The model under review builds one solid part; all positions refer to its coordinate system, in mm. Round coordinates to 2 decimals unless told otherwise and drop trailing zeros. Answer as a JSON object with one key per item and string values. Group by question number.
1) Insertion check: pin 1 Ø8 at (y, z) = (4, 57) entering from -X; pin 2 Ø3 at (y, z) = (4, 68) entering from +X; pin 3 Ø4 at (y, z) = (3, 47.5) entering from -X. Each pin has a flat end and moves straight along its axis. Give the tip position at first contact, or say it passes through.
2) To check wall thickness, follow probe 1 along Z at (x, y) = (0.5, -13); probe 2 along Z at (x, y) = (-1.5, 2); probe 3 along Z at (x, y) = (0, -3.5). State the ranges of each line that lie inside material, in increasing order. Write a range as [from, to].
3) We need section A-A, the plane x = 19. Count the separate pieces of the cut face and the enclosed holes in it, then the cut area to 3 significant figures.
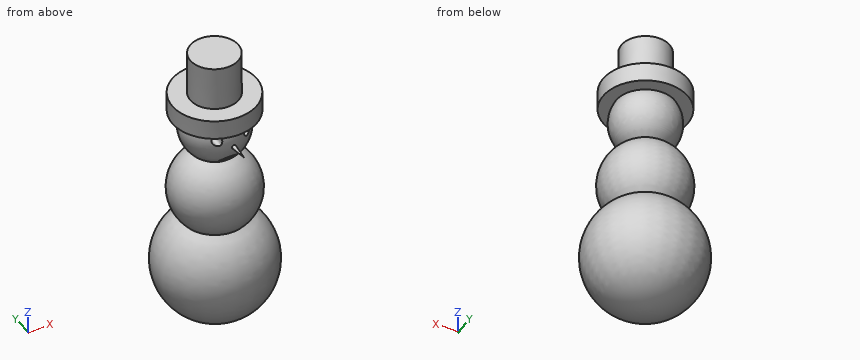
from build123d import *

# Parameters (mm, degrees)
F4_R     = 2.9313934917
F6_DEPTH = 25.4


with BuildPart() as f1:
    # F0 (on Front) → F1 (revolve)
    with BuildSketch(Plane.XZ):
        with BuildLine():
            ThreePointArc((-8.6470126601, 59.8095870837), (-21.4016690603, 44.0535851857), (-15.695191047, 24.6018766648))
            ThreePointArc((-15.695191047, 24.6018766648), (-28.0136061915, -8.1749144079), (0, -29.1820382673))
            Line((0, -29.1820382673), (-0.3967727534, 114.0140891075))
            Line((-0.3967727534, 114.0140891075), (-12.4211851507, 114.0140891075))
            Line((-12.4211851507, 114.0140891075), (-12.4211851507, 92.0014604926))
            Line((-12.4211851507, 92.0014604926), (-21.4189756662, 92.0014604926))
            Line((-21.4189756662, 92.0014604926), (-21.4189756662, 82.3283791542))
            Line((-21.4189756662, 82.3283791542), (-14.9194911479, 82.3283791542))
            ThreePointArc((-14.9194911479, 82.3283791542), (-16.2978226924, 69.8114756975), (-8.6470126601, 59.8095870837))
        make_face()
    revolve(axis=Axis((-0.1983863767, 0, 42.4160254201), (0.0027708237, 0, -0.9999961613)))

    # F4 (on Front) → F5 section 0
    with BuildSketch(Plane.XZ, mode=Mode.PRIVATE) as f5_s0:
        with Locations((0, 72.6552978158)):
            Circle(F4_R)
    loft([Vertex(0, -25.4, 72.6552978158), f5_s0.sketch])

    # F3 (on offset) → F6 (cut)
    with BuildSketch(Plane.XZ.offset(25.4)):
        with BuildLine():
            add(Edge.make_bspline(
                [(-8.0269714817, 79.5348510146), (-8.6846337437, 79.4264052352), (-9.8414942897, 78.1450545351), (-9.497142748, 75.3585343357), (-5.8915269462, 74.1267113958), (-5.1057227017, 77.4839777864), (-5.9214182567, 78.8940297376), (-7.3670372691, 79.6436714293), (-8.0269714817, 79.5348510146)],
                knots=[0, 0, 0, 0, 0.1593701812, 0.3340862186, 0.5188256822, 0.6983768822, 0.8400792609, 1, 1, 1, 1], degree=3))
        make_face()
        with BuildLine():
            add(Edge.make_bspline(
                [(8.3799511194, 78.3284604549), (7.624080444, 78.6857899226), (5.8447857804, 78.4029369239), (5.6907424207, 76.3172160457), (7.506583602, 73.9429964977), (10.3601830594, 76.0452757725), (9.1859243667, 77.9474455529), (8.3799511194, 78.3284604549)],
                knots=[0, 0, 0, 0, 0.1981616253, 0.3732706853, 0.5804624626, 0.7887033142, 1, 1, 1, 1], degree=3))
        make_face()
        with BuildLine():
            Line((3.1171578952, 62.8545942359), (4.2782197706, 63.3692070842))
            ThreePointArc((4.2782197706, 63.3692070842), (-0.4267061595, 66.4302188327), (-5.1316320896, 63.3692070842))
            Line((-5.1316320896, 63.3692070842), (-3.9705702142, 62.8545942359))
            ThreePointArc((-3.9705702142, 62.8545942359), (-0.4267061595, 65.1602223516), (3.1171578952, 62.8545942359))
        make_face()
    extrude(amount=-F6_DEPTH, mode=Mode.SUBTRACT)


solid = f1.part
Here are the results:
{
 "1": {"pin 1": "stops at x = -17", "pin 2": "stops at x = 15.24", "pin 3": "stops at x = -20.9"},
 "2": {"probe 1": "z = [-26.08, 57.14], [63.91, 65.05], [66.35, 92.04]", "probe 2": "z = [-29.07, 114.02]", "probe 3": "z = [-28.96, 65.14], [66.41, 114.02]"},
 "3": {"separate pieces": "3", "enclosed holes": "0", "area": "2,000 mm^2"}
}
